```python
from build123d import *

# Parameters (mm, degrees)
F0_R     = 2.00025
F1_DEPTH = 9.525
F2_W     = 55.258708
F2_H     = 2.54
F2_W_2   = 16.308993
F3_DEPTH = 152.40108
F4_W     = 16.884602
F4_H     = 12.087842
F4_W_2   = 13.239063
F4_H_2   = 22.832589
F4_W_3   = 22.832591
F4_H_3   = 36.455397
F4_W_4   = 24.841385
F4_H_4   = 50.653815
F5_DEPTH = 25.4


with BuildPart() as f1:
    # F0 (on Top) → F1 (new body)
    with BuildSketch(Plane.XY):
        with BuildLine():
            Line((12.7, 0), (12.699599, 63.600882))
            ThreePointArc((12.699599, 63.600882), (6.63067, 74.33163), (-5.686228, 74.855915))
            Line((-5.686228, 74.855915), (-131.355282, 11.929858))
            ThreePointArc((-131.355282, 11.929858), (-139.554552, -1.916565), (-127.59746, -12.685939))
            Line((-127.59746, -12.685939), (-0.59746, -12.685939))
            ThreePointArc((-0.59746, -12.685939), (8.766478, -9.189063), (12.7, 0))
        make_face()
        with Locations((-127, 0)):
            Circle(F0_R, mode=Mode.SUBTRACT)
        with Locations((0, 63.5)):
            Circle(F0_R, mode=Mode.SUBTRACT)
    extrude(amount=F1_DEPTH)

    # F2 (on face) → F3 (cut, through all)
    with BuildSketch(Plane(origin=(12.7, 8e-05, 0), x_dir=(-6e-06, 1, 0), z_dir=(1, 6e-06, 0))):
        with Locations((27.629274, 8.255)):
            Rectangle(F2_W, F2_H)
        with Locations((27.629274, 1.27)):
            Rectangle(F2_W, F2_H)
        with Locations((-8.154576, 1.27)):
            Rectangle(F2_W_2, F2_H)
        with Locations((-8.154576, 8.255)):
            Rectangle(F2_W_2, F2_H)
    extrude(amount=-F3_DEPTH, mode=Mode.SUBTRACT)

    # F4 (on face) → F5 (cut)
    with BuildSketch(Plane.XY.offset(6.985)):
        with Locations((-105.618868, 6.043921)):
            Rectangle(F4_W, F4_H)
        with Locations((-78.46919, 11.416294)):
            Rectangle(F4_W_2, F4_H_2)
        with Locations((-47.961781, 18.227698)):
            Rectangle(F4_W_3, F4_H_3)
        with Locations((-12.420692, 25.326907)):
            Rectangle(F4_W_4, F4_H_4)
    extrude(amount=-F5_DEPTH, mode=Mode.SUBTRACT)


solid = f1.part
```
The model under review builds one solid part; all positions refer to its coordinate system, in mm. A direction names the side the tool comes from. Round coordinates to 2 decimals unless told otherwise and drop trailing zeros. Order: outer loops, then holes, each group sorted by start corner. A loop starts at its lowest first (then second) coordinate and runs counter-clockwise, first axis right, second up.
Item 1: Add section C-C, the plane x = -111. State the section outline as (y, z) points (3 decimals).
Working result:
outline: (-12.686, 2.54) - (0, 2.54) - (0, 6.985) - (-12.686, 6.985) - close; (12.088, 2.54) - (22.122, 2.54) - (22.122, 6.985) - (12.088, 6.985) - close
Item 2: Add section B-B, the plane y = 31.5. State the section outline as (x, z) points (3 decimals).
Working result:
outline: (-92.272, 2.54) - (-59.378, 2.54) - (-59.378, 6.985) - (-92.272, 6.985) - close; (-36.545, 2.54) - (-24.841, 2.54) - (-24.841, 6.985) - (-36.545, 6.985) - close; (0, 2.54) - (12.7, 2.54) - (12.7, 6.985) - (0, 6.985) - close
Item 3: Add section D-D, the plane y = 8.5. State the section outline as (x, z) points (3 decimals).
Working result:
outline: (-136.436, 2.54) - (-114.061, 2.54) - (-114.061, 6.985) - (-136.436, 6.985) - close; (-97.177, 2.54) - (-85.089, 2.54) - (-85.089, 6.985) - (-97.177, 6.985) - close; (-71.85, 2.54) - (-59.378, 2.54) - (-59.378, 6.985) - (-71.85, 6.985) - close; (-36.545, 2.54) - (-24.841, 2.54) - (-24.841, 6.985) - (-36.545, 6.985) - close; (0, 2.54) - (12.7, 2.54) - (12.7, 6.985) - (0, 6.985) - close
Item 4: Machinability: for faces 1 (the flat face through (-13, 50.654, 5)), 2 (the flat face through (-10, 64, 0)), 3 (the flat face through (-62, 14, 2.54)), which of the approach directions +Z, -Z, +X, -X, +Y, -Y give a long, thin tool a straight path to every point of the face, cutting with its end or side? Answer none if there is none.
Working result:
face 1: +Z, -Z
face 2: -Z, +X, -X, +Y, -Y
face 3: -Z, +X, -X, -Y
Item 5: Add section A-A, the plane z = 5. State the section outline as (x, y) points, and give its area (3 significant figures).
Working result:
outline: (-131.36, 11.93) arc R12.7 ccw to (-127.6, -12.69) - (-0.6, -12.69) arc R12.7 ccw to (12.7, 0) - (12.7, 63.6) arc R12.7 ccw to (-5.69, 74.86) - close; hole circle Ø4 at (-127, 0); hole (-114.06, 0) - (-97.18, 0) - (-97.18, 12.09) - (-114.06, 12.09) - close; hole (-85.09, 0) - (-71.85, 0) - (-71.85, 22.83) - (-85.09, 22.83) - close; hole (-59.38, 0) - (-36.55, 0) - (-36.55, 36.46) - (-59.38, 36.46) - close; hole (-24.84, 0) - (0, 0) - (0, 50.65) - (-24.84, 50.65) - close; hole circle Ø4 at (0, 63.5)
area: 6,130 mm2
Item 6: To check wall thickness, follow probe 1 along Y at (x, z) = (0, 7.25); probe 2 along X at (y, z) = (12.5, 4); probe 3 along X at (y, z) = (31.5, 6.75). State the ranges of each line that lie inside material, in increasing order.
Working result:
probe 1: y = 55.26 to 61.5, 65.5 to 76.2
probe 2: x = -130.22 to -85.09, -71.85 to -59.38, -36.55 to -24.84, 0 to 12.7
probe 3: x = -92.27 to -59.38, -36.55 to -24.84, 0 to 12.7
Item 7: Draft analysis for pull direction X (two halves, no side actions). For faces 4 (the flat face through (-85.089, 11, 5)), 5 (the cylindrical face through (-139.59, -1.68, 4.73)), 6 (the cylindrical face through (6.78, 74.24, 4.7)), state which applies: released by +X, released by -X, zero draft, split by the parting line, or undercut.
Working result:
face 4: undercut
face 5: released by -X
face 6: split by the parting line
Item 8: For pin 1 (5 mm diameter, centred on y = 14.5, z = 4, fed in from -X); pin 2 (1.3 mm diameter, centred on x = -107.5, z = 5, fed in from -Y); pin 3 (3 mm diameter, centred on x = -92, y = 20.5, fed in from +Z) (3 decimals), all flat-tipped, find the tip position at first contact; note any pin that passes through.
Working result:
pin 1: stops at x = -131.22
pin 2: stops at y = -12.69
pin 3: stops at z = 6.985
